Read the model definition and answer for the solid it produces. Units are mm, in the model's axes. A direction names the side the tool comes from. Round coordinates to 2 decimals unless told otherwise and drop trailing zeros. Write each loop counter-clockwise with the first axis right and the second up, starting at its lowest first coordinate (ties: lowest second). Pieces come first, ordered by that corner, then holes.
from build123d import *

# Parameters (mm, degrees)
F2_W     = 8.886791
F2_H     = 11.736567
F2_W_2   = 7.621294
F3_DEPTH = 20


with BuildPart() as f1:
    # F0 (on Front) → F1 (revolve)
    with BuildSketch(Plane.XZ):
        Polygon((0, 43.325846), (0, 0), (3, 0), (3, 40), (4.52552, 40), (8.148538, 44.563168), (6.648163, 46.424412), (3, 43.325846), align=None)
    revolve(axis=Axis((0, 0, 21.662923), (0, 0, 1)))

    # F2 (on Right) → F3 (cut, symmetric)
    with BuildSketch(Plane.YZ):
        with Locations((-7.005405, 47.46977)):
            Rectangle(F2_W, F2_H)
        with Locations((6.248638, 47.46977)):
            Rectangle(F2_W_2, F2_H)
    extrude(amount=F3_DEPTH, both=True, mode=Mode.SUBTRACT)


solid = f1.part
Q1. Which of the six approach directions +Z, -Z, +X, -X, +Y, -Y give full straight-line access (tool end or side, diameter ignored) to faces 1 (the flat face through (0, 0, 0)), 2 (the flat face through (0, -4, 41.601)), 3 (the conical face through (-4.39, -0.1, 44.51)), 4 (the flat face through (0, 4, 41.601)), 5 (the cylindrical face through (-3, 0, 20))?
Verdict:
face 1: -Z, +X, -X, +Y, -Y
face 2: +Z, +X, -X, -Y
face 3: +Z
face 4: +Z, +X, -X, +Y
face 5: -Z
Q2. Section A-A (y = 0) is taken. Determine the outline of the cut face in (x, z).
Verdict:
outline: (-8.15, 44.56) - (-4.53, 40) - (-3, 40) - (-3, 0) - (3, 0) - (3, 40) - (4.53, 40) - (8.15, 44.56) - (6.65, 46.42) - (3, 43.33) - (-3, 43.33) - (-6.65, 46.42) - close
Q3. Straight lines are drawn through the part: probe 1 along Y at (x, z) = (-0.25, 7); probe 2 along Z at (x, y) = (-0.25, 2.25). For each, find the intervals that lie inside material, in ascending order.
Verdict:
probe 1: y = -2.99 to 2.99
probe 2: z = 0 to 43.33
Q4. Flat-ended cylindrical pins translate along their axes: pin 1 Ø2.5 at (x, y) = (-1, -4) entering from +Z; pin 2 Ø1 at (x, z) = (-2, 12.5) entering from +Y; pin 3 Ø4 at (y, z) = (2.5, 35.5) entering from +X. Find the tip coordinate at first contact, or state that the pin passes through.
Verdict:
pin 1: stops at z = 41.6
pin 2: stops at y = 2.6
pin 3: stops at x = 2.96
Q5. Section B-B (x = 0) is taken. Determine the outline of the cut face in (y, z), then the cut area to 3 significant figures.
Verdict:
outline: (-5.8, 41.6) - (-4.53, 40) - (-3, 40) - (-3, 0) - (3, 0) - (3, 40) - (4.53, 40) - (5.8, 41.6) - (2.44, 41.6) - (2.44, 43.33) - (-2.56, 43.33) - (-2.56, 41.6) - close
area: 265 mm2
Q6. Determine the mould class of faces 6 (the flat face through (-3, -1, 40)), 7 (the conical face through (4.39, -0.23, 44.51)), 8 (the flat face through (0, -2.562, 43)) for opening direction Y: pulls with the +Y half, pulls with the -Y half, needs draft (parallel to the pull), parting line crosses it, or undercut.
Verdict:
face 6: needs draft
face 7: undercut
face 8: pulls with the -Y half
Q7. Section C-C (z = 10.5) is taken. Determine the outline of the cut face in (x, y).
Verdict:
outline: circle Ø6 at (0, 0)
